The drawing under review shows one solid part. Ordinate dimensions are in mm from its lowest x, y, z. A direction names the side the tool comes from. Give positions to 0.01 mm unless a question says otherwise; leave off trailing zeros. Order: outer loops, then holes, each group sorted by start corner. A loop starts at its lowest first (then second) coordinate and runs counter-clockwise, first axis right, second up. Notation, with made-up numbers: (14.5, 11.5) - (24.5, 11.5) arc R19 cw to (24.5, 20.5) - close; hole circle Ø11 at (-6, -12.75). An arc over 180 degrees is marked (long way). Answer as a JSON object with one key per item and string values. Group by question number.
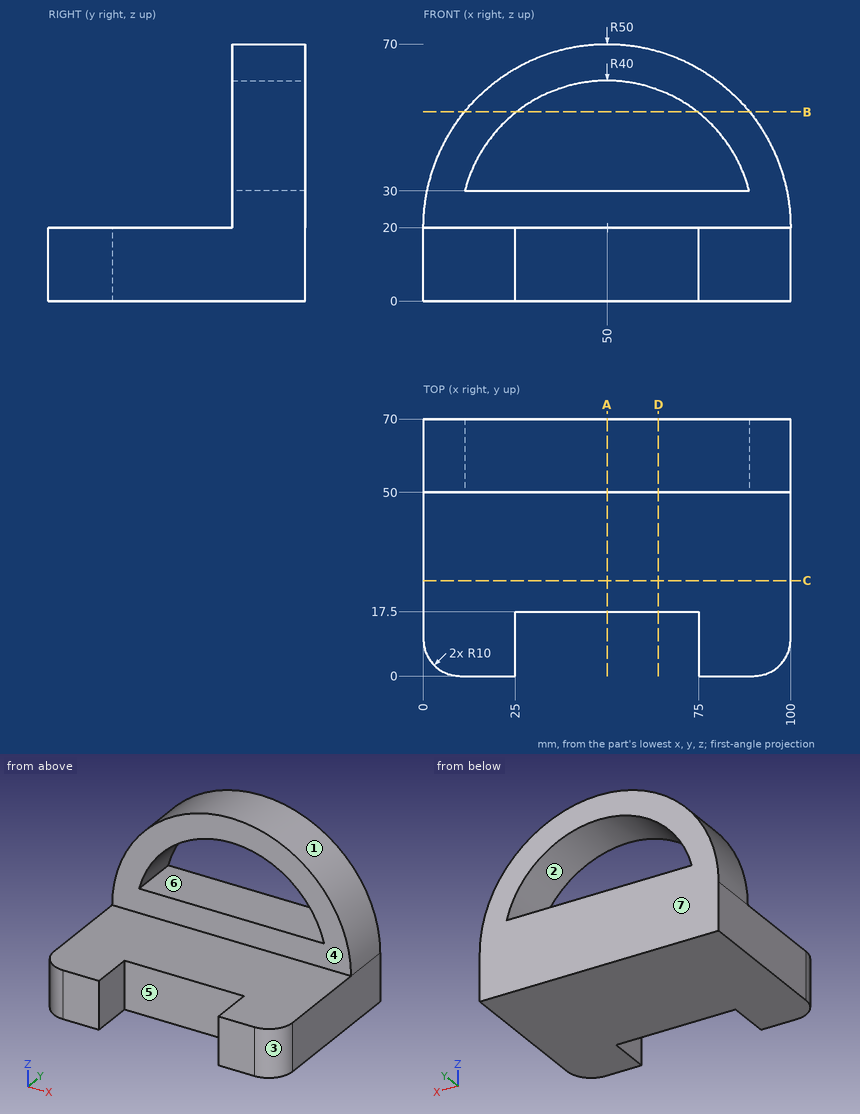
1) Consider section C-C (y = 26). Give the boundary of the cut face in (x, z).
2) Consider section A-A (x = 50). Give the boundary of the cut face in (y, z).
3) Mouldability with a two-part tool opening along Z and no side actions: class the marked faces 1, 2 and 3 as released by +Z, released by -Z, zero draft, split by the parting line, or undercut.
4) Consider section B-B (z = 51.5). Give the boundary of the cut face in (x, y), plus the area to 3 significant figures.
5) For pin 1 (6 mm diameter, centred on x = 55.5, y = 61, fed in from +Z); pin 2 (8 mm diameter, centred on x = 12.5, z = 24.5, fed in from -Y); pin 3 (1.5 mm diameter, centred on x = 19, z = 31.5, fed in from +Y); pin 4 (3 mm diameter, centred on x = 14.5, y = 30.5, fed in from +Z), all flat-tipped, find the tip position at first contact; note any pin that passes through.
6) Consider section D-D (x = 64). Give the boundary of the cut face in (y, z), plus the area to 3 significant figures.
7) For the marked faces 4, 5, 6 and 7, list the 3-axis set-ups (+Z, -Z, +X, -X, +Y, -Y) from which the entire face can be reached by the end or side of a thin tool; tool diameter is ignored.
8) For line 1 (Z direction, x = 27, y = 36.5); line 2 (X direction, y = 10, z = 7); line 3 (Y direction, x = 22.5, z = 20.5), list the stretches that pass through material, from the lowest coordinate up.
Result set:
{
 "1": {"outline": "(0, 0) - (100, 0) - (100, 20) - (0, 20) - close"},
 "2": {"outline": "(17.5, 0) - (70, 0) - (70, 30) - (50, 30) - (50, 20) - (17.5, 20) - close; (50, 60) - (70, 60) - (70, 70) - (50, 70) - close"},
 "3": {"face 1": "released by +Z", "face 2": "undercut", "face 3": "zero draft"},
 "4": {"outline": "(11.17, 50) - (25.35, 50) - (25.35, 70) - (11.17, 70) - close; (74.65, 50) - (88.83, 50) - (88.83, 70) - (74.65, 70) - close", "area": "567 mm2"},
 "5": {"pin 1": "stops at z = 69.94", "pin 2": "stops at y = 50", "pin 3": "passes through", "pin 4": "stops at z = 20"},
 "6": {"outline": "(17.5, 0) - (70, 0) - (70, 30) - (50, 30) - (50, 20) - (17.5, 20) - close; (50, 57.47) - (70, 57.47) - (70, 68) - (50, 68) - close", "area": "1,460 mm2"},
 "7": {"face 4": "+Z, +X, -X, -Y", "face 5": "+Z, -Z, -Y", "face 6": "+Y, -Y", "face 7": "+Z, -Z, +X, -X, +Y"},
 "8": {"line 1": "z = 0 to 20", "line 2": "x = 0 to 25, 75 to 100", "line 3": "y = 50 to 70"}
}
